Input: part model. Units: mm. Frame: model coordinates. A direction names the side the tool comes from. Coordinates: 2 decimals unless noted, no trailing zeros. Write each loop counter-clockwise with the first axis right and the second up, starting at its lowest first coordinate (ties: lowest second). Pieces come first, ordered by that corner, then holes. Notation, with made-up numbers: (-22, 31) -> (31, 31) arc R16 ccw to (31, 35) -> close; hole circle Ø8 at (43, -22). An arc over 180 degrees is marked (long way). Use one line per item in the form item = value. Start each with the question number.
(1) Ray query, line 1 along Z through (x, y) = (-30, -17); line 2 along X through (y, z) = (-3, 13.5); line 3 along X through (y, z) = (-27, -6). Return the intervals inside material, ascending.
(2) Set-up query: faces 1 (the face through (-7, -45, 12.7)), 2 (the face through (13, -26, 12.7)), 3 (the face through (32, -26, -6.35)). Return all of +Z, -Z, +X, -X, +Y, -Y with unobstructed straight access to the full face (end or side cutting, diameter ignored); none if empty.
(3) Pull-direction query (Y, two-part tool) for faces 4 (the face through (-1, -50.8, 0)), 5 (the face through (-44.45, -25, -13)), 6 (the face through (-21, -26, 0)); classes: released by +Y, released by -Y, zero draft, split by the parting line, or undercut.
(4) First-contact query: pin 1 (6.5 mm diameter, centred on x = -35.5, y = -16.5, fed in from +Z); pin 2 (10 mm diameter, centred on y = -31, z = 9, fed in from -X); pin 3 (12.5 mm diameter, centred on x = -11, y = -47.5, fed in from +Z). Flat tips, straight axial feed; report the tip coordinate or a pass-through.
(5) Cut plane C-C on y = -20.5. Return the cut outline in (x, z), plus the area to 3 significant figures.
(6) Cut plane B-B on z = 2.5. Return the cut outline in (x, y), plus the area to 3 significant figures.
(7) Cut plane A-A on x = -6.35. Return the cut outline in (y, z), plus the area to 3 significant figures.
(8) Cut plane D-D on y = -5. Return the cut outline in (x, z), plus the area to 3 significant figures.
```python
from build123d import *

# Parameters (mm, degrees)
F0_W      = 88.9
F0_H      = 38.1
F1_DEPTH  = 50.8
F2_W      = 25.4
F2_H      = 25.4
F3_DEPTH  = 50.801
F4_W      = 12.7
F4_H      = 25.4
F5_DEPTH  = 50.801
F6_W      = 25.4
F6_H      = 6.35
F7_DEPTH  = 50.801
F9_W      = 50.733156
F9_H      = 26.686712
F10_DEPTH = 12.7
F8_R      = 7.757908
F11_DEPTH = 50.801


with BuildPart() as f1:
    # F0 (on Front) → F1 (new body)
    with BuildSketch(Plane.XZ):
        Rectangle(F0_W, F0_H)
    extrude(amount=F1_DEPTH)

    # F2 (on face) → F3 (cut, through all)
    with BuildSketch(Plane.XZ.offset(50.8)):
        with Locations((31.75, 6.35)):
            Rectangle(F2_W, F2_H)
    extrude(amount=-F3_DEPTH, mode=Mode.SUBTRACT)

    # F4 (on face) → F5 (cut, through all)
    with BuildSketch(Plane(origin=(0, 0, 0), x_dir=(-1, 0, 0), z_dir=(0, 1, 0))):
        with Locations((38.1, 6.35)):
            Rectangle(F4_W, F4_H)
    extrude(amount=-F5_DEPTH, mode=Mode.SUBTRACT)

    # F6 (on face) → F7 (cut, through all)
    with BuildSketch(Plane.XZ.offset(50.8)):
        with Locations((-6.35, 15.875)):
            Rectangle(F6_W, F6_H)
    extrude(amount=-F7_DEPTH, mode=Mode.SUBTRACT)

    # F9 (on face) → F10 (cut)
    with BuildSketch(Plane.XY.offset(12.7)):
        with Locations((-6.366711, -26.043356)):
            Rectangle(F9_W, F9_H)
    extrude(amount=-F10_DEPTH, mode=Mode.SUBTRACT)

    # F8 (on face) → F11 (cut, through all)
    with BuildSketch(Plane.XZ.offset(50.8)):
        with Locations((-6.35, -6.35)):
            Circle(F8_R)
    extrude(amount=-F11_DEPTH, mode=Mode.SUBTRACT)


solid = f1.part
```
Values:
q1.line_1 = -19.05 to 0, 12.7 to 19.05
q1.line_2 = -31.75 to -19.05, 6.35 to 19.05
q1.line_3 = -31.75 to -14.1, 1.4 to 19.05
q2.face_1 = +Z, +Y, -Y
q2.face_2 = none
q2.face_3 = +Z, +X, +Y, -Y
q3.face_4 = released by -Y
q3.face_5 = zero draft
q3.face_6 = undercut
q4.pin_1 = -6.35
q4.pin_2 = -31.75
q4.pin_3 = 12.7
q5.outline = (-44.45, -19.05) -> (44.45, -19.05) -> (44.45, -6.35) -> (19.05, -6.35) -> (19.05, 19.05) -> (6.35, 19.05) -> (6.35, 12.7) -> (19, 12.7) -> (19, 0) -> (-1.89, 0) arc R7.76 cw (long way) to (-10.81, 0) -> (-31.73, 0) -> (-31.73, 12.7) -> (-19.05, 12.7) -> (-19.05, 19.05) -> (-31.75, 19.05) -> (-31.75, -6.35) -> (-44.45, -6.35) -> close
q5.area = 1,430 mm2
q6.outline = (-31.75, -50.8) -> (19.05, -50.8) -> (19.05, 0) -> (-31.75, 0) -> close; hole (-31.73, -39.39) -> (19, -39.39) -> (19, -12.7) -> (-31.73, -12.7) -> close
q6.area = 1,230 mm2
q7.outline = (-50.8, -19.05) -> (0, -19.05) -> (0, -14.11) -> (-50.8, -14.11) -> close; (-50.8, 1.41) -> (-39.39, 1.41) -> (-39.39, 12.7) -> (-50.8, 12.7) -> close; (-12.7, 1.41) -> (0, 1.41) -> (0, 12.7) -> (-12.7, 12.7) -> close
q7.area = 523 mm2
q8.outline = (-44.45, -19.05) -> (44.45, -19.05) -> (44.45, -6.35) -> (19.05, -6.35) -> (19.05, 19.05) -> (6.35, 19.05) -> (6.35, 12.7) -> (-19.05, 12.7) -> (-19.05, 19.05) -> (-31.75, 19.05) -> (-31.75, -6.35) -> (-44.45, -6.35) -> close; hole circle Ø15.52 at (-6.35, -6.35)
q8.area = 2,070 mm2
